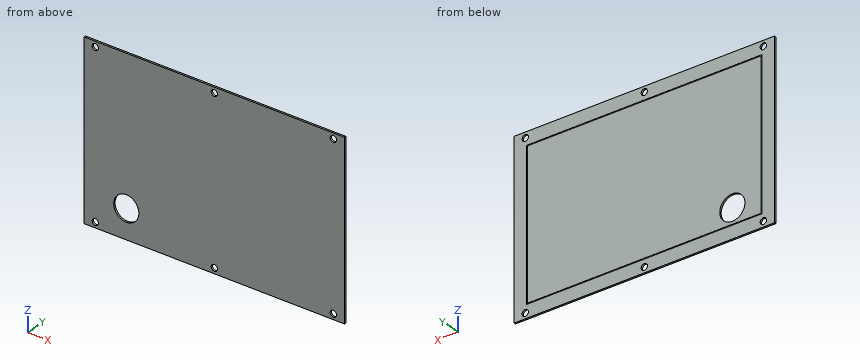
```python
from build123d import *

# Parameters (mm, degrees)
F0_W     = 290
F0_H     = 190
F1_DEPTH = 2
F3_D     = 7
F4_W     = 262
F4_H     = 162
F4_W_2   = 260
F4_H_2   = 160
F5_DEPTH = 0.2
F7_D     = 28


with BuildPart() as f1:
    # F0 (on Front) → F1 (new body)
    with BuildSketch(Plane.XZ):
        with Locations((36.382314, 28.64574)):
            Rectangle(F0_W, F0_H)
    extrude(amount=F1_DEPTH)

    # F3 (through all)
    with Locations(Plane.XZ.offset(2)):
        with Locations((-96.117686, 117.64574), (36.382314, 117.64574), (168.882314, 117.64574), (168.882314, -60.35426), (36.382314, -60.35426), (-96.117686, -60.35426)):
            Hole(F3_D / 2)

    # F4 (on face) → F5 (cut)
    with BuildSketch(Plane.XZ):
        with Locations((36.382314, 28.64574)):
            Rectangle(F4_W, F4_H)
        with Locations((36.382314, 28.64574)):
            Rectangle(F4_W_2, F4_H_2, mode=Mode.SUBTRACT)
    extrude(amount=F5_DEPTH, mode=Mode.SUBTRACT)

    # F7 (through all)
    with Locations(Plane.XZ.offset(2)):
        with Locations((-61.617686, -34.35426)):
            Hole(F7_D / 2)


solid = f1.part
```
Check sheet for the modelled part. Datum: model origin and axes. Units: mm. Give positions to 0.01 mm unless a question says otherwise; leave off trailing zeros. Write each loop counter-clockwise with the first axis right and the second up, starting at its lowest first coordinate (ties: lowest second). Pieces come first, ordered by that corner, then holes. Notation, with made-up numbers: (-11, 34) -> (-6, 34) arc R20 cw to (-6, 61) -> close; hole circle Ø5 at (47.25, 63). An arc over 180 degrees is marked (long way). Use CSV: the item, a comma, the result in double quotes. Start each with the question number.
Q1. Cross-section at A-A on z = -26. Enter the section's corners in (x, y), and give its area (3 significant figures).
Q2. Cross-section at B-B on x = -55.5. Enter the section's corners in (y, z).
Q3. Scan lines: line 1 along X through (y, z) = (-0.1, 55); line 2 along Z through (x, y) = (5, -0.1); line 3 along Y through (x, z) = (-94, -4.5). Record each from-to range of solid material in increasing order.
Q4. Depth check by flat-ended pin: P1, Ø8, axis at x = 168.88, z = 117.65, coming from the +Y side. Enter the tip coordinate at first touch or a pass-through.
Q5. Cross-section at C-C on y = -1.2. Enter the section's corners in (x, z).
Working result:
1,outline,"(-108.62, -2) -> (-72.85, -2) -> (-72.85, 0) -> (-93.62, 0) -> (-93.62, -0.2) -> (-94.62, -0.2) -> (-94.62, 0) -> (-108.62, 0) -> close; (-50.38, -2) -> (181.38, -2) -> (181.38, 0) -> (167.38, 0) -> (167.38, -0.2) -> (166.38, -0.2) -> (166.38, 0) -> (-50.38, 0) -> close"
1,area,"535 mm^2"
2,outline,"(-2, -66.35) -> (0, -66.35) -> (0, -52.35) -> (-0.2, -52.35) -> (-0.2, -51.35) -> (0, -51.35) -> (0, -46.95) -> (-2, -46.95) -> close; (-2, -21.76) -> (0, -21.76) -> (0, 108.65) -> (-0.2, 108.65) -> (-0.2, 109.65) -> (0, 109.65) -> (0, 123.65) -> (-2, 123.65) -> close"
3,line 1,"x = -108.62 to -94.62, -93.62 to 166.38, 167.38 to 181.38"
3,line 2,"z = -66.35 to -52.35, -51.35 to 108.65, 109.65 to 123.65"
3,line 3,"y = -2 to -0.2"
4,P1,"stops at y = 0"
5,outline,"(-108.62, -66.35) -> (181.38, -66.35) -> (181.38, 123.65) -> (-108.62, 123.65) -> close; hole circle Ø7 at (-96.12, -60.35); hole circle Ø7 at (-96.12, 117.65); hole circle Ø28 at (-61.62, -34.35); hole circle Ø7 at (36.38, -60.35); hole circle Ø7 at (36.38, 117.65); hole circle Ø7 at (168.88, -60.35); hole circle Ø7 at (168.88, 117.65)"
